Work out the finished part from the listing and answer in its coordinate system (mm). A direction names the side the tool comes from. Coordinates: 2 decimals unless noted, no trailing zeros. Loops run counter-clockwise (first coordinate to the right, second up) from the corner with the lowest first, then second, coordinate; pieces in that order, holes last. Notation, with made-up numbers: (23, -6) -> (76, -6) arc R24 cw to (76, 14) -> close; hole circle Ø10 at (-37.75, -3). An arc over 180 degrees is marked (long way). Use a Markdown table: item, result.
from build123d import *

# Parameters (mm, degrees)
SKETCH004_W     = 30
SKETCH004_H     = 16
PAD003_DEPTH    = 2
SKETCH005_R     = 3.4
POCKET001_DEPTH = 20
PAD004_DEPTH    = 25
SKETCH006_R     = 12.2
POCKET002_DEPTH = 30
SKETCH007_R     = 1.2
SKETCH007_R_2   = 1.1
POCKET003_DEPTH = 5
SKETCH008_R     = 1.4
POCKET004_DEPTH = 50


with BuildPart() as part:
    # Sketch004 → Pad003 (new body)
    with BuildSketch(Plane.XY.offset(30)):
        with Locations((0, -5.045388)):
            Rectangle(SKETCH004_W, SKETCH004_H)
    extrude(amount=PAD003_DEPTH)

    # Sketch005 (on Face3 of Pad) → Pocket001 (cut)
    with BuildSketch(Plane.XY.offset(30)):
        Circle(SKETCH005_R)
    extrude(amount=POCKET001_DEPTH, mode=Mode.SUBTRACT)

    # Sketch004 → Pad004 (join)
    with BuildSketch(Plane.XY.offset(30)):
        with Locations((0, -5.045388)):
            Rectangle(SKETCH004_W, SKETCH004_H)
    extrude(amount=-PAD004_DEPTH)

    # Sketch006 → Pocket002 (cut)
    with BuildSketch(Plane.XY):
        Circle(SKETCH006_R)
    extrude(amount=POCKET002_DEPTH, mode=Mode.SUBTRACT)

    # Sketch007 (on Face5 of Pocket002) → Pocket003 (cut)
    with BuildSketch(Plane.XY.offset(32)):
        with Locations((-7.016269, 0)):
            Circle(SKETCH007_R)
        with Locations((7.016269, 0)):
            Circle(SKETCH007_R_2)
    extrude(amount=-POCKET003_DEPTH, mode=Mode.SUBTRACT)

    # Sketch008 (on Face5 of Pocket003) → Pocket004 (cut)
    with BuildSketch(Plane.XY.offset(32)):
        with Locations((-10, -10.95175)):
            Circle(SKETCH008_R)
        with Locations((10, -10.95175)):
            Circle(SKETCH008_R)
    extrude(amount=-POCKET004_DEPTH, mode=Mode.SUBTRACT)


solid = part.part
Q1. Section D-D on z = 19.5 is taken. Determine the outline of the cut face in (x, y).
Solved:
| item | result |
|---|---|
| outline | (-15, -13.05) -> (15, -13.05) -> (15, 2.95) -> (11.84, 2.95) arc R12.2 cw (long way) to (-11.84, 2.95) -> (-15, 2.95) -> close; hole circle Ø2.8 at (-10, -10.95); hole circle Ø2.8 at (10, -10.95) |
Q2. Determine the mould class of faces 3 (the flat face through (0, -5, 32)), 4 (the cylindrical face through (-11.4, -10.9, 18.7)), 5 (the flat face through (-15, -5, 19)), 6 (the flat face through (15, -5, 19)) for opening direction X: pulls with the +X half, pulls with the -X half, needs draft (parallel to the pull), parting line crosses it, or undercut.
Solved:
| item | result |
|---|---|
| face 3 | needs draft |
| face 4 | undercut |
| face 5 | pulls with the -X half |
| face 6 | pulls with the +X half |
Q3. Consider line 1 (Z direction, x = 8.5, y = -8.25); line 2 (X direction, y = 0.75, z = 23); line 3 (X direction, y = -1.25, z = 7). Determine where each line is inside the solid, lowest interval first. Write a range as [from, to].
Solved:
| item | result |
|---|---|
| line 1 | [30, 32] |
| line 2 | [-15, -12.18], [12.18, 15] |
| line 3 | [-15, -12.14], [12.14, 15] |
Q4. For faces 1 (the flat face through (1, -12.7, 5)), 2 (the cylindrical face through (-0.31, -12.196, 17.325)), determine the directions among +Z, -Z, +X, -X, +Y, -Y from which every point of the face is accessible in a straight line to the end or side of a thin tool.
Solved:
| item | result |
|---|---|
| face 1 | -Z, +X, -X, +Y, -Y |
| face 2 | -Z |
Q5. Section A-A on y = 0 is taken. Determine the outline of the cut face in (x, z), and give its area (3 significant figures).
Solved:
| item | result |
|---|---|
| outline | (-15, 5) -> (-12.2, 5) -> (-12.2, 30) -> (-8.22, 30) -> (-8.22, 32) -> (-15, 32) -> close; (-5.82, 30) -> (-3.4, 30) -> (-3.4, 32) -> (-5.82, 32) -> close; (3.4, 30) -> (5.92, 30) -> (5.92, 32) -> (3.4, 32) -> close; (8.12, 30) -> (12.2, 30) -> (12.2, 5) -> (15, 5) -> (15, 32) -> (8.12, 32) -> close |
| area | 177 mm² |
Q6. Section B-B on x = 9.5 is taken. Determine the outline of the cut face in (y, z), and give its area (3 significant figures).
Solved:
| item | result |
|---|---|
| outline | (-13.05, 5) -> (-12.26, 5) -> (-12.26, 32) -> (-13.05, 32) -> close; (-9.64, 5) -> (-7.65, 5) -> (-7.65, 30) -> (2.95, 30) -> (2.95, 32) -> (-9.64, 32) -> close |
| area | 96.2 mm² |
Q7. Section C-C on y = -11.5 is taken. Determine the outline of the cut face in (x, z), and give its area (3 significant figures).
Solved:
| item | result |
|---|---|
| outline | (-15, 5) -> (-11.29, 5) -> (-11.29, 32) -> (-15, 32) -> close; (-8.71, 5) -> (-4.07, 5) -> (-4.07, 30) -> (4.07, 30) -> (4.07, 5) -> (8.71, 5) -> (8.71, 32) -> (-8.71, 32) -> close; (11.29, 5) -> (15, 5) -> (15, 32) -> (11.29, 32) -> close |
| area | 467 mm² |
Q8. Given pin 1 Ø2.5 at (x, y) = (7.02, 0) entering from -Z; pin 2 Ø2.5 at (x, y) = (-10, -10.95) entering from +Z, each flat-ended and moving along its own axis, determine where each tip first touches the part or whether it passes through.
Solved:
| item | result |
|---|---|
| pin 1 | z = 30 |
| pin 2 | through |
